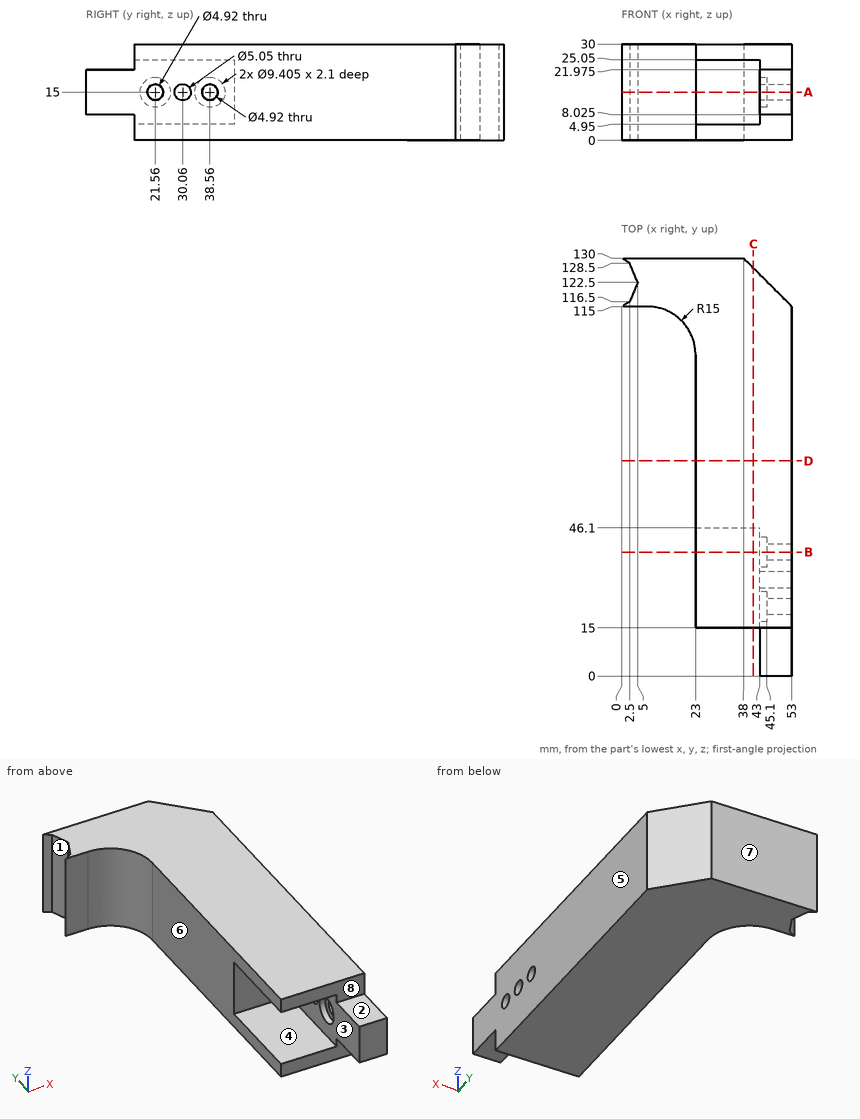
Geometry check sheet. Reference: drawing and pictorial views, mm from the part's lowest x, y, z. A direction names the side the tool comes from. Give positions to 0.01 mm unless a question says otherwise; leave off trailing zeros. Write each loop counter-clockwise with the first axis right and the second up, starting at its lowest first coordinate (ties: lowest second). Pieces come first, ordered by that corner, then holes.
Item 1: Cross-section at B-B (y = 38.56). Enter the section's corners in (x, z), and give its area (3 significant figures).
Item 2: Cross-section at C-C (x = 41). Enter the section's corners in (y, z), and give its area (3 significant figures).
Item 3: Draft check along Z on the marked faces 1, 2 and 3. Enter one of: released by +Z, released by -Z, zero draft, split by the parting line, or undercut.
Item 4: Scan lines: L1, parallel to Z at x = 30, y = 17.5; L2, parallel to Y at x = 50, z = 15 (3 decimals); L3, parallel to Y at x = 50.5, z = 15 (3 decimals). Record each from-to range of solid material in increasing order.
Item 5: Access from +Z, -Z, +X, -X, +Y, -Y to the whole of each face (thin tool, end or side, straight path). Record for the marked faces 4, 5, 6, 7 and 8.
Item 6: Cross-section at D-D (y = 67). Enter the section's corners in (x, z), and give its area (3 significant figures).
Item 7: Cross-section at A-A (z = 15). Count the separate pieces of the cut face and the enclosed holes in it, and give its area (3 significant figures).
Item 8: Gauge pin test, flat ends, axial feed: pin 1 (11 mm diameter, centred on x = 48.5, y = 4, fed in from -Z) (3 decimals); pin 2 (5 mm diameter, centred on x = 17, z = 9, fed in from -Y); pin 3 (6 mm diameter, centred on y = 30.06, z = 15, fed in from -X); pin 4 (8 mm diameter, centred on x = 42.5, z = 16, fed in from -Y). Record the tip position at first contact, or that the pin passes through.
Report:
1. outline: (23, 0) - (53, 0) - (53, 12.54) - (45.1, 12.54) - (45.1, 10.3) - (43, 10.3) - (43, 4.95) - (23, 4.95) - close; (23, 25.05) - (43, 25.05) - (43, 19.7) - (45.1, 19.7) - (45.1, 17.46) - (53, 17.46) - (53, 30) - (23, 30) - close
1. area: 439 mm2
2. outline: (15, 0) - (127, 0) - (127, 30) - (15, 30) - (15, 25.05) - (46.1, 25.05) - (46.1, 4.95) - (15, 4.95) - close
2. area: 2,730 mm2
3. face 1: zero draft
3. face 2: released by +Z
3. face 3: undercut
4. L1: z = 0 to 4.95, 25.05 to 30
4. L2: y = 0 to 19.1, 24.02 to 27.535, 32.585 to 36.1, 41.02 to 118
4. L3: y = 0 to 19.1, 24.02 to 27.535, 32.585 to 36.1, 41.02 to 117.5
5. face 4: -X, -Y
5. face 5: +Z, -Z, +X, +Y, -Y
5. face 6: +Z, -Z, -X, -Y
5. face 7: +Z, -Z, +X, -X, +Y
5. face 8: +Z, +X, -X, -Y
6. outline: (23, 0) - (53, 0) - (53, 30) - (23, 30) - close
6. area: 900 mm2
7. separate pieces: 4
7. enclosed holes: 0
7. area: 3,040 mm2
8. pin 1: stops at z = 8.025
8. pin 2: stops at y = 109.63
8. pin 3: stops at x = 43
8. pin 4: stops at y = 0
